```python
from build123d import *

# Parameters (mm, degrees)
F1_DEPTH = 1.25222
F3_DEPTH = 1.016
F4_W     = 12.7
F4_H     = 7.112
F5_DEPTH = 1.016
F6_W     = 15.24
F6_H     = 2.032
F7_DEPTH = 25.4
F8_R     = 0.508


with BuildPart() as f1:
    # F0 (on Front) → F1 (new body)
    with BuildSketch(Plane.XZ):
        with BuildLine():
            Line((27.6567419321, -7.07644), (29.3056013183, -7.07644))
            ThreePointArc((29.3056013183, -7.07644), (29.7092433479, -5.4653384255), (29.845, -3.81))
            Line((29.845, -3.81), (29.845, 3.81))
            ThreePointArc((29.845, 3.81), (26.8692048969, 10.9942048969), (19.685, 13.97))
            Line((19.685, 13.97), (-19.685, 13.97))
            ThreePointArc((-19.685, 13.97), (-26.8692048969, 10.9942048969), (-29.845, 3.81))
            Line((-29.845, 3.81), (-29.845, -3.81))
            ThreePointArc((-29.845, -3.81), (-29.7092433479, -5.4653384255), (-29.3056013183, -7.07644))
            Line((-29.3056013183, -7.07644), (-27.6567419321, -7.07644))
            ThreePointArc((-27.6567419321, -7.07644), (-28.2480586179, -5.230243154), (-28.448, -3.302))
            Line((-28.448, -3.302), (-28.448, 3.302))
            ThreePointArc((-28.448, 3.302), (-25.6953895296, 9.9473895296), (-19.05, 12.7))
            Line((-19.05, 12.7), (19.05, 12.7))
            ThreePointArc((19.05, 12.7), (25.6953895296, 9.9473895296), (28.448, 3.302))
            Line((28.448, 3.302), (28.448, -3.302))
            ThreePointArc((28.448, -3.302), (28.2480586179, -5.230243154), (27.6567419321, -7.07644))
        make_face()
        with BuildLine():
            Line((-19.685, -13.97), (19.685, -13.97))
            ThreePointArc((19.685, -13.97), (25.1077661576, -12.4018104728), (28.8565313119, -8.18134))
            Line((28.8565313119, -8.18134), (27.0820884684, -8.18134))
            ThreePointArc((27.0820884684, -8.18134), (23.6579478448, -11.4928009779), (19.05, -12.7))
            Line((19.05, -12.7), (-19.05, -12.7))
            ThreePointArc((-19.05, -12.7), (-23.6579478448, -11.4928009779), (-27.0820884684, -8.18134))
            Line((-27.0820884684, -8.18134), (-28.8565313119, -8.18134))
            ThreePointArc((-28.8565313119, -8.18134), (-25.1077661576, -12.4018104728), (-19.685, -13.97))
        make_face()
        with BuildLine():
            Line((-29.3056013183, -7.07644), (-28.8565313119, -8.18134))
            Line((-28.8565313119, -8.18134), (-27.0820884684, -8.18134))
            ThreePointArc((-27.0820884684, -8.18134), (-27.3877377194, -7.6384194588), (-27.6567419321, -7.07644))
            Line((-27.6567419321, -7.07644), (-29.3056013183, -7.07644))
        make_face()
        with BuildLine():
            Line((27.0820884684, -8.18134), (28.8565313119, -8.18134))
            Line((28.8565313119, -8.18134), (29.3056013183, -7.07644))
            Line((29.3056013183, -7.07644), (27.6567419321, -7.07644))
            ThreePointArc((27.6567419321, -7.07644), (27.3877377194, -7.6384194588), (27.0820884684, -8.18134))
        make_face()
        with BuildLine():
            Line((-27.6567419321, -7.07644), (27.6567419321, -7.07644))
            ThreePointArc((27.6567419321, -7.07644), (28.2480586179, -5.230243154), (28.448, -3.302))
            Line((28.448, -3.302), (28.448, 3.302))
            ThreePointArc((28.448, 3.302), (25.6953895296, 9.9473895296), (19.05, 12.7))
            Line((19.05, 12.7), (-19.05, 12.7))
            ThreePointArc((-19.05, 12.7), (-25.6953895296, 9.9473895296), (-28.448, 3.302))
            Line((-28.448, 3.302), (-28.448, -3.302))
            ThreePointArc((-28.448, -3.302), (-28.2480586179, -5.230243154), (-27.6567419321, -7.07644))
        make_face()
        with BuildLine():
            Line((-27.0820884684, -8.18134), (27.0820884684, -8.18134))
            ThreePointArc((27.0820884684, -8.18134), (27.3877377194, -7.6384194588), (27.6567419321, -7.07644))
            Line((27.6567419321, -7.07644), (-27.6567419321, -7.07644))
            ThreePointArc((-27.6567419321, -7.07644), (-27.3877377194, -7.6384194588), (-27.0820884684, -8.18134))
        make_face()
        with BuildLine():
            ThreePointArc((19.05, -12.7), (23.6579478448, -11.4928009779), (27.0820884684, -8.18134))
            Line((27.0820884684, -8.18134), (-27.0820884684, -8.18134))
            ThreePointArc((-27.0820884684, -8.18134), (-23.6579478448, -11.4928009779), (-19.05, -12.7))
            Line((-19.05, -12.7), (19.05, -12.7))
        make_face()
    extrude(amount=F1_DEPTH)

    # F2 (on face) → F3 (join)
    with BuildSketch(Plane.XZ.offset(1.25222)):
        with BuildLine():
            Line((-19.05, -12.7), (19.05, -12.7))
            ThreePointArc((19.05, -12.7), (23.6579478448, -11.4928009779), (27.0820884684, -8.18134))
            Line((27.0820884684, -8.18134), (-27.0820884684, -8.18134))
            ThreePointArc((-27.0820884684, -8.18134), (-23.6579478448, -11.4928009779), (-19.05, -12.7))
        make_face()
        with BuildLine():
            Line((-27.6567419321, -7.07644), (27.6567419321, -7.07644))
            ThreePointArc((27.6567419321, -7.07644), (28.2480586179, -5.230243154), (28.448, -3.302))
            Line((28.448, -3.302), (28.448, 3.302))
            ThreePointArc((28.448, 3.302), (25.6953895296, 9.9473895296), (19.05, 12.7))
            Line((19.05, 12.7), (-19.05, 12.7))
            ThreePointArc((-19.05, 12.7), (-25.6953895296, 9.9473895296), (-28.448, 3.302))
            Line((-28.448, 3.302), (-28.448, -3.302))
            ThreePointArc((-28.448, -3.302), (-28.2480586179, -5.230243154), (-27.6567419321, -7.07644))
        make_face()
    extrude(amount=F3_DEPTH)

    # F4 (on face) → F5 (cut)
    with BuildSketch(Plane.XZ.offset(2.26822)):
        with Locations((-3.429, -3.52044)):
            Rectangle(F4_W, F4_H)
        with Locations((10.795, -3.52044)):
            Rectangle(F4_W, F4_H)
    extrude(amount=-F5_DEPTH, mode=Mode.SUBTRACT)

    # F6 (on face) → F7 (cut)
    with BuildSketch(Plane.XZ.offset(2.26822)):
        with Locations((-10.795, -9.19734)):
            Rectangle(F6_W, F6_H)
    extrude(amount=-F7_DEPTH, mode=Mode.SUBTRACT)

    # F8
    f8_edges = [f1.edges().sort_by_distance(p)[0] for p in [
        (17.145, -1.76022, -7.07644),
        (17.145, -1.76022, 0.03556),
        (4.445, -1.76022, -7.07644),
        (4.445, -1.76022, 0.03556),
        (-9.779, -1.76022, 0.03556),
        (2.921, -1.76022, 0.03556),
        (2.921, -1.76022, -7.07644),
        (-9.779, -1.76022, -7.07644),
        (-3.175, -1.13411, -10.21334),
        (-18.415, -0.62611, -8.18134),
        (-18.415, -1.13411, -10.21334),
        (-3.175, -0.62611, -8.18134),
    ]]
    fillet(f8_edges, radius=F8_R)


solid = f1.part
```
Verification items for the finished model (mm, model axes). A direction names the side the tool comes from. Coordinates: 2 decimals unless noted, no trailing zeros. Write each loop counter-clockwise with the first axis right and the second up, starting at its lowest first coordinate (ties: lowest second). Pieces come first, ordered by that corner, then holes. Notation, with made-up numbers: M 50,10.5 L 68,10.5 A13 cw 68,28.5 Z; hole C 61,72.5 d3. An arc over 180 degrees is marked long. Answer as a JSON object with one key per item and string values. Group by question number.
(1) Cross-section at B-B, the plane y = -0.5. Record the cut outline in (x, z) (3 decimals).
(2) Cross-section at A-A, the plane x = -12. Record the cut outline in (y, z).
(3) Release check for a two-part mould opening along Z. For faces 1 (the face through (0, -1, 13.97)), 2 (the face through (0, -2.268, -10)), 3 (the face through (-3.175, -1, -9)) record: +Z half, -Z half, draft (parallel to the pull), parting line (faces both ways), or undercut.
(4) Cross-section at D-D, the plane z = -1.5. Record the cut outline in (x, y) (3 decimals), and give its area (3 significant figures).
(5) Material ranges on line 1 (Z direction, x = 12, y = -1.4); line 2 (Z direction, x = -8.5, y = -1.05); line 3 (X direction, y = -1.3, z = -5.5) (3 decimals), recorded low to high.
(6) Tool access check on faces 4 (the face through (0, -2, 12.7)), 5 (the face through (-11, -1, -10.213)), 6 (the face through (12, -2, -8.181)), 7 (the face through (11, -2, 0.036)), 8 (the face through (23.599, -1.753, -11.526)). Record the directions out of +Z, -Z, +X, -X, +Y, -Y that give a thin tool (end or side, any length) a straight path to the whole face; none if there is none.
(7) Gauge pin test, flat ends, axial feed: pin 1 (0.5 mm diameter, centred on y = -2, z = -0.5, fed in from -X); pin 2 (1.1 mm diameter, centred on x = -3.5, y = -2, fed in from +Z); pin 3 (0.8 mm diameter, centred on x = -16, y = -2, fed in from -Z). Record the tip position at first contact, or that the pin passes through.
(8) Cross-section at C-C, the plane x = 0. Record the cut outline in (y, z), and give its area (3 significant figures).
Reply:
{
 "1": {"outline": "M -29.845,-3.81 A10.16 ccw -29.306,-7.076 L -28.857,-8.181 A10.16 ccw -19.685,-13.97 L 19.685,-13.97 A10.16 ccw 28.857,-8.181 L 29.306,-7.076 A10.16 ccw 29.845,-3.81 L 29.845,3.81 A10.16 ccw 19.685,13.97 L -19.685,13.97 A10.16 ccw -29.845,3.81 Z; hole M -18.415,-9.705 A0.508 ccw -17.907,-10.213 L -3.683,-10.213 A0.508 ccw -3.175,-9.705 L -3.175,-8.689 A0.508 ccw -3.683,-8.181 L -17.907,-8.181 A0.508 ccw -18.415,-8.689 Z"},
 "2": {"outline": "M -2.27,-12.7 L -1.25,-12.7 L -1.25,-13.97 L 0,-13.97 L 0,-10.21 L -2.27,-10.21 Z; M -2.27,-7.08 L -1.25,-7.08 L -1.25,-8.18 L 0,-8.18 L 0,13.97 L -1.25,13.97 L -1.25,12.7 L -2.27,12.7 Z"},
 "3": {"face 1": "+Z half", "face 2": "draft", "face 3": "undercut"},
 "4": {"outline": "M -29.845,-1.252 L -28.448,-1.252 L -28.448,-2.268 L -9.779,-2.268 L -9.779,-1.252 L 2.921,-1.252 L 2.921,-2.268 L 4.445,-2.268 L 4.445,-1.252 L 17.145,-1.252 L 17.145,-2.268 L 28.448,-2.268 L 28.448,-1.252 L 29.845,-1.252 L 29.845,0 L -29.845,0 Z", "area": "107 mm²"},
 "5": {"line 1": "-12.7 to -8.18, 0.04 to 12.7", "line 2": "-13.97 to -10.21, -8.18 to 13.97", "line 3": "-28.187 to -9.779, 2.921 to 4.445, 17.145 to 28.187"},
 "6": {"face 4": "+Z, +X, -X, -Y", "face 5": "+Y, -Y", "face 6": "+X, -X, -Y", "face 7": "-Y", "face 8": "-Z, +X, -Y"},
 "7": {"pin 1": "x = -28.45", "pin 2": "z = 12.7", "pin 3": "z = -12.7"},
 "8": {"outline": "M -2.27,-12.7 L -1.25,-12.7 L -1.25,-13.97 L 0,-13.97 L 0,13.97 L -1.25,13.97 L -1.25,12.7 L -2.27,12.7 L -2.27,0.04 L -1.25,0.04 L -1.25,-8.18 L -2.27,-8.18 Z", "area": "52.4 mm²"}
}
